Design review of the part built by this model. Coordinates are the model's own, in mm. A direction names the side the tool comes from. Give positions to 0.01 mm unless a question says otherwise; leave off trailing zeros. Order: outer loops, then holes, each group sorted by start corner. A loop starts at its lowest first (then second) coordinate and runs counter-clockwise, first axis right, second up. Notation, with made-up numbers: M 40,-22.5 L 46,-22.5 A9 ccw 46,-6.5 Z; hole C 54.5,72 d2. An arc over 180 degrees is marked long. Answer as a JSON object with one key per item and string values.
from build123d import *

# Parameters (mm, degrees)
F0_W     = 41
F0_H     = 20
F1_DEPTH = 27
F2_W     = 7
F2_H     = 18
F2_R     = 2
F3_DEPTH = 2.5
F4_DEPTH = 12
F5_R     = 2.95
F6_DEPTH = 3.5


with BuildPart() as f1:
    # F0 (on Top) → F1 (new body)
    with BuildSketch(Plane.XY):
        Rectangle(F0_W, F0_H)
    extrude(amount=F1_DEPTH)

    # F2 (on face) → F3 (join)
    with BuildSketch(Plane.XY.offset(27)):
        Polygon((20.5, 9), (20.5, 10), (-20.5, 10), (-20.5, 9), (-20.5, -9), (-20.5, -10), (20.5, -10), (20.5, -9), align=None)
        with Locations((24, 0)):
            Rectangle(F2_W, F2_H)
        with Locations((25, -5)):
            Circle(F2_R, mode=Mode.SUBTRACT)
        with Locations((25, 5)):
            Circle(F2_R, mode=Mode.SUBTRACT)
        with Locations((-24, 0)):
            Rectangle(F2_W, F2_H)
        with Locations((-25, -5)):
            Circle(F2_R, mode=Mode.SUBTRACT)
        with Locations((-25, 5)):
            Circle(F2_R, mode=Mode.SUBTRACT)
    extrude(amount=F3_DEPTH)

    # F2 (on face) → F4 (join)
    with BuildSketch(Plane.XY.offset(27)):
        Polygon((20.5, 9), (20.5, 10), (-20.5, 10), (-20.5, 9), (-20.5, -9), (-20.5, -10), (20.5, -10), (20.5, -9), align=None)
    extrude(amount=F4_DEPTH)

    # F5 (on face) → F6 (join)
    with BuildSketch(Plane.XY.offset(39)):
        with Locations((-10.95, 0)):
            Circle(F5_R)
    extrude(amount=F6_DEPTH)


solid = f1.part
(1) We need section B-B (x = -10.95). Write out the cut boundary in (y, z), plus the area to 3 significant figures.
Checked values:
{"outline": "M -10,0 L 10,0 L 10,39 L 2.95,39 L 2.95,42.5 L -2.95,42.5 L -2.95,39 L -10,39 Z", "area": "801 mm^2"}
(2) To check wall thickness, follow L1, parallel to Y at x = -25, z = 28; L2, parallel to X at y = -2.5, z = 20.5; L3, parallel to Z at x = 4.5, y = -7.25. State the ranges of each line that lie inside material, in increasing order. Write a range as from..to.
Checked values:
{"L1": "y = -9..-7, -3..3, 7..9", "L2": "x = -20.5..20.5", "L3": "z = 0..39"}
(3) Draft analysis for pull direction Y (two halves, no side actions). For faces 1 (the cylindrical face through (23, 5, 28)), 2 (the flat face through (-11, 0, 42.5)), 3 (the cylindrical face through (-26.6, -6.2, 28.2)), 4 (the cylindrical face through (-8.136, 0.886, 40.726)), state which applies: +Y half, -Y half, draft (parallel to the pull), parting line (faces both ways), or undercut.
Checked values:
{"face 1": "undercut", "face 2": "draft", "face 3": "undercut", "face 4": "parting line"}
(4) Tool access review of faces 5 (the flat face through (24, 9, 28)), 6 (the flat face through (24, -9, 28)), 7 (the flat face through (-24, 0, 29.5)), 8 (the flat face through (-24, 9, 28)): name each direction out of +Z, -Z, +X, -X, +Y, -Y from which nothing blocks a thin tool from reaching the whole face with its end or side.
Checked values:
{"face 5": "+Z, -Z, +X, +Y", "face 6": "+Z, -Z, +X, -Y", "face 7": "+Z, -X, +Y, -Y", "face 8": "+Z, -Z, -X, +Y"}
(5) We need section A-A (y = -5). Write out the cut boundary in (x, z), plus the area to 3 significant figures.
Checked values:
{"outline": "M -27.5,27 L -27,27 L -27,29.5 L -27.5,29.5 Z; M -23,27 L -20.5,27 L -20.5,0 L 20.5,0 L 20.5,27 L 23,27 L 23,29.5 L 20.5,29.5 L 20.5,39 L -20.5,39 L -20.5,29.5 L -23,29.5 Z; M 27,27 L 27.5,27 L 27.5,29.5 L 27,29.5 Z", "area": "1,610 mm^2"}
(6) Insertion check: pin 1 (2 mm diameter, centred on x = 1.5, y = 6, fed in from -Z); pin 2 (1 mm diameter, centred on y = 2.5, z = 14, fed in from -X); pin 3 (6 mm diameter, centred on x = 9.5, y = 3, fed in from +Z); pin 4 (5 mm diameter, centred on x = 25, y = -5, fed in from +Z). Each pin has a flat end and moves straight along its axis. Give the tip position at first contact, or say it passes through.
Checked values:
{"pin 1": "stops at z = 0", "pin 2": "stops at x = -20.5", "pin 3": "stops at z = 39", "pin 4": "stops at z = 29.5"}
(7) We need section D-D (z = 24.5). Write out the cut boundary in (x, y), plus the area to 3 significant figures.
Checked values:
{"outline": "M -20.5,-10 L 20.5,-10 L 20.5,10 L -20.5,10 Z", "area": "820 mm^2"}
(8) We need section C-C (y = 0). Write out the cut boundary in (x, z), plus the area to 3 significant figures.
Checked values:
{"outline": "M -27.5,27 L -20.5,27 L -20.5,0 L 20.5,0 L 20.5,27 L 27.5,27 L 27.5,29.5 L 20.5,29.5 L 20.5,39 L -8,39 L -8,42.5 L -13.9,42.5 L -13.9,39 L -20.5,39 L -20.5,29.5 L -27.5,29.5 Z", "area": "1,650 mm^2"}
